from build123d import *

# Parameters (mm, degrees)
F1_DEPTH = 21
F2_R     = 1
F3_R     = 0.5


with BuildPart() as f1:
    # F0 (on Right) → F1 (new body)
    with BuildSketch(Plane.YZ):
        Polygon((-40, 3), (-40, 0), (0, 0), (0, -20), (3, -20), (3, 3), align=None)
    extrude(amount=F1_DEPTH)

    # F2
    f2_edges = [f1.edges().sort_by_distance(p)[0] for p in [
        (10.5, 3, 3),
        (21, -40, 1.5),
        (0, -40, 1.5),
        (21, 1.5, -20),
        (0, 1.5, -20),
    ]]
    fillet(f2_edges, radius=F2_R)

    # F3
    f3_edges = [f1.edges().sort_by_distance(p)[0] for p in [
        (10.5, 0, 0),
    ]]
    fillet(f3_edges, radius=F3_R)


solid = f1.part
Source: CAD feature listing. Evaluate the final solid. Frame: model axes, mm. A direction names the side the tool comes from. Round coordinates to 2 decimals unless told otherwise and drop trailing zeros. Loops run counter-clockwise (first coordinate to the right, second up) from the corner with the lowest first, then second, coordinate; pieces in that order, holes last.
Q1. Section B-B, the plane y = -33. Return loops of the section in (x, z).
Q2. First-contact query: P1, Ø8, axis at y = -23.5, z = -3, coming from the -X side; P2, Ø4, axis at y = -32.5, z = -3.5, coming from the -X side; P3, Ø2, axis at x = 6.5, y = -19, coming from the -Z side; P4, Ø1.5, axis at x = 18, z = -16, coming from the -Y side. Flat tips, straight axial feed; report the tip coordinate or a pass-through.
Q3. Section A-A, the plane x = 12.25. Return loops of the section in (y, z).
Q4. Ray query, line 1 (Z direction, x = 1.5, y = -13). Return the intervals inside material, ascending.
Q5. Access query for faces 1 (the face through (0.301, 1.521, -19.715)), 2 (the face through (10, 0, -10)). Directions: +Z, -Z, +X, -X, +Y, -Y. A direction counts if a zero-diameter tool reaches every point of the face in a straight line with its end or side. Return the directions, or none.
Solutions:
1. outline: (0, 0) - (21, 0) - (21, 3) - (0, 3) - close
2. P1: stops at x = 0
2. P2: passes through
2. P3: stops at z = 0
2. P4: stops at y = 0
3. outline: (-40, 0) - (-0.5, 0) arc R0.5 cw to (0, -0.5) - (0, -20) - (3, -20) - (3, 2) arc R1 ccw to (2, 3) - (-40, 3) - close
4. line 1: z = 0 to 3
5. face 1: -Z, -X, +Y, -Y
5. face 2: -Z, +X, -X, -Y
